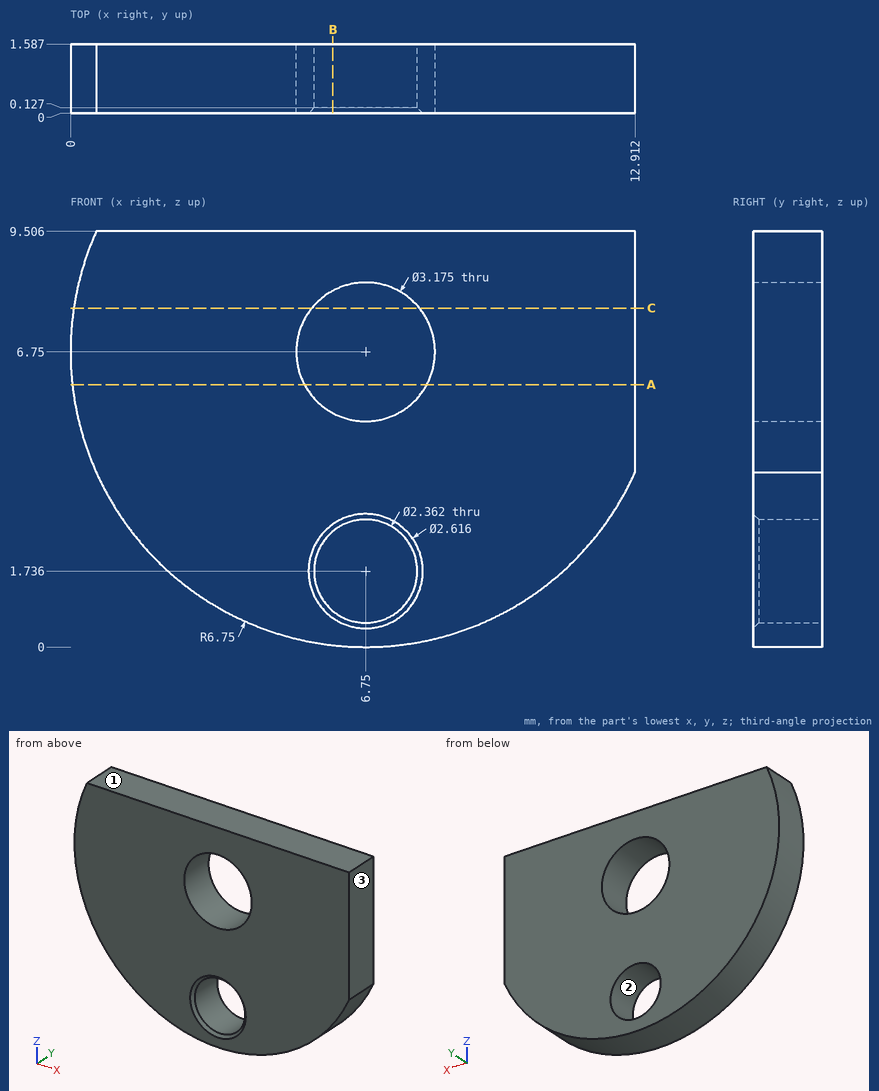
Verification items for this drawing (mm, ordinates from the low corner). Give positions to 0.01 mm unless a question says otherwise; leave off trailing zeros. Loops run counter-clockwise (first coordinate to the right, second up) from the corner with the lowest first, then second, coordinate; pieces in that order, holes last.
(1) Section check C-C on z = 7.75. Record the cut outline in (x, y) (1 decimal).
From the geometry:
outline: (0.1, 0) - (5.5, 0) - (5.5, 1.6) - (0.1, 1.6) - close; (8, 0) - (12.9, 0) - (12.9, 1.6) - (8, 1.6) - close
(2) Release check for a two-part mould opening along X. For the marked faces 1, 2 and 3 record: released by +X, released by -X, zero draft, split by the parting line, or undercut.
From the geometry:
face 1: zero draft
face 2: undercut
face 3: released by +X
(3) Thickness scan on L1, parallel to Z at x = 7.25, y = 0.75 (1 decimal); L2, parallel to X at y = 0.25, z = 6.75; L3, parallel to X at y = 0.4, z = 1.5 (1 decimal). Record the ranges inside material, lowest first.
From the geometry:
L1: z = 0 to 0.7, 2.8 to 5.2, 8.3 to 9.5
L2: x = 0 to 5.16, 8.34 to 12.91
L3: x = 2.5 to 5.6, 7.9 to 11
(4) Section check A-A on z = 6. Record the cut outline in (x, y), then the cut area to 3 significant figures.
From the geometry:
outline: (0.04, 0) - (5.35, 0) - (5.35, 1.59) - (0.04, 1.59) - close; (8.15, 0) - (12.91, 0) - (12.91, 1.59) - (8.15, 1.59) - close
area: 16.0 mm2
(5) Section check B-B on x = 6. Count the separate pieces of the cut face and the enclosed holes in it.
From the geometry:
separate pieces: 3
enclosed holes: 0
